Autodesk Inventor part; units mm, degrees
ref_plane "Work Plane1" through (-20.8033, -6.3, -5.9) normal (0, 0, 1) x (1, 0, 0)
ref_plane "YZ Plane" through (0, 0, 0) normal (1, 0, 0) x (0, 1, 0)
ref_plane "XZ Plane" through (0, 0, 0) normal (0, 1, 0) x (-1, 0, 0)
sketch "Sketch1" plane through (0, 0, 0) normal (0, 0, 1) x (1, 0, 0)
  line L0 (0.8467, -0.7217) -> (0.8467, 0.7217) construction
  line L1 (0.8467, 0.7217) -> (2.0967, 1.4434) construction
  line L2 (2.0967, 1.4434) -> (3.3467, 0.7217) construction
  line L3 (3.3467, 0.7217) -> (3.3467, -0.7217) construction
  line L4 (3.3467, -0.7217) -> (2.0967, -1.4434) construction
  line L5 (2.0967, -1.4434) -> (0.8467, -0.7217) construction
  circle A0 centre (2.0967, 0) radius 2.45 construction
  line L6 (4.8467, -1.5877) -> (3.4717, -2.3816) construction
  line L7 (15.0967, 3) -> (15.0967, -3) construction
  line L8 (-10.9033, 3) -> (-10.9033, -3) construction
  line L9 (-0.6533, 0) -> (-0.6533, 1.5877) construction
  circle A1 centre (2.0967, 0) radius 5
  circle A2 centre (2.0967, 0) radius 1.7
  line L10 (-10.9033, -3) -> (15.0967, -3)
  line L11 (-10.9033, 3) -> (15.0967, 3)
  circle A3 centre (2.0967, 0) radius 2.75
  circle A4 centre (2.0967, 0) radius 6.5
  point P0 (0.4719, -0.5)
  point P1 (3.7215, -0.5)
  dimension "d10" = 5.5
  dimension "d13" = 13
ref_plane "Work Plane1" through (-20.8033, -6.3, -5.9) normal (0, 0, 1) x (1, 0, 0)
extrude "Extrusion1" add sketch "Sketch1" against normal blind 5 contours A1 L10 L11 | A1 L11 A4 L10 | L11 A1 | A1 L11 A4 | L10 A4 A1 | A1 L10 | A1 L10 A4 L11
sketch "Sketch2" plane through (2.0967, 0, 0) normal (0, 0, 1) x (1, 0, 0)
  line L0 (-2, 1.5) -> (2, 1.5) construction
  arc A0 (2.5, 0) -> (2, 1.5) centre (0, 0) ccw construction
  arc A1 (-2, 1.5) -> (-2.5, 0) centre (0, 0) ccw construction
  line L1 (2, -1.5) -> (-2, -1.5) construction
  arc A2 (-2.5, 0) -> (2.5, 0) centre (0, 0) ccw construction
  line L2 (2.0248, 1.55) -> (-2.0248, 1.55) construction
  arc A3 (-2.0248, 1.55) -> (-2.55, 0) centre (0, 0) ccw construction
  arc A4 (-2.55, 0) -> (2.55, 0) centre (0, 0) ccw construction
  arc A5 (2.55, 0) -> (2.0248, 1.55) centre (0, 0) ccw construction
  line L3 (-2.0248, 1.55) -> (2.0248, 1.55) construction
  line L4 (-2.0248, 1.55) -> (2.0248, 1.55)
  line L5 (-2.0248, -1.55) -> (2.0248, -1.55)
  arc A6 (-2.0248, 1.55) -> (-2.0248, -1.55) centre (0, 0) ccw
  arc A7 (2.0248, -1.55) -> (2.0248, 1.55) centre (0, 0) ccw
  circle A8 centre (0, 0) radius 6.5
  point P0 (-2.0967, 0)
  dimension "d11" = 3.1
  dimension "d12" = 2.55
extrude "Extrusion2" add sketch "Sketch2" along normal blind 7
chamfer "Chamfer1" distance 1.2 angle 45 4 edges at (2.0967, 1.55, 7) (-0.4533, 0, 7) (2.0967, -1.55, 7) (4.6467, 0, 7)
sketch "Sketch3" plane through (0, 0, 0) normal (0, 1, 0) x (-1, 0, 0)
  line L0 (-4.6467, 0) -> (-4.6467, 5.8)
  line L1 (0.4533, 0) -> (0.4533, 5.8)
  line L2 (-8.5967, -5) -> (4.4033, -5)
  circle A0 centre (-2.0967, -2.5) radius 1.25
  line L3 (-8.5967, -5) -> (4.4033, -5)
  point P0 (0, 0)
  point P1 (-8.5967, 0)
  point P2 (4.4033, 0)
  dimension "d14" = 2.5
  dimension "d15" = 2.5
extrude "Extrusion3" cut sketch "Sketch3" against normal blind 10
pattern_circular "Circular Pattern1" count 2 over 360 about axis through (2.0967, 0, 0) along (0, 0, -1) of "Extrusion3"
sketch "Sketch4" plane through (0.0718, -1.55, 0) normal (0, 1, 0) x (1, 0, 0)
  line L0 (0, -5.8) -> (4.0497, -5.8)
  line L1 (-4.4752, -7) -> (8.5248, -7)
  line L2 (8.5248, 5) -> (-4.4752, 5)
  line L3 (4.0497, -5.8) -> (0, -5.8)
  line L4 (4.0497, 0) -> (4.0497, -5.8)
  line L5 (0, 0) -> (0, -5.8)
  circle A0 centre (2.0248, -2.0248) radius 2.0248
  line L6 (0, 0) -> (4.0497, 0)
  point P0 (-0.0718, 0)
  point P1 (3.2748, 2.5)
  point P2 (0.7748, 2.5)
hole "Hole1" at (2.0967, -1.55, 2.0248) direction (0, -1, 0) diameter 2.5 end through all both
properties part number "30_Coupling_Screw_28BYJ_M3_v2"
Geometry check sheet. Reference: the model listing, model coordinates, mm. A direction names the side the tool comes from. Give positions to 0.01 mm unless a question says otherwise; leave off trailing zeros. Loops run counter-clockwise (first coordinate to the right, second up) from the corner with the lowest first, then second, coordinate; pieces in that order, holes last.
(1) Section check A-A on y = 0. Record the cut outline in (x, z), then the cut area to 3 significant figures.
From the geometry:
outline: (-4.4, -5) - (-0.65, -5) - (-0.65, 0) - (-0.45, 0) - (-0.45, 5.8) - (-1.65, 7) - (-4.4, 7) - close; (4.65, 0) - (4.85, 0) - (4.85, -5) - (8.6, -5) - (8.6, 7) - (5.85, 7) - (4.65, 5.8) - close
area: 91.4 mm2
(2) Depth check by flat-ended pin: pin 1 Ø4 at (y, z) = (-3, -1.5) entering from +X; pin 2 Ø3 at (y, z) = (-4.5, 1) entering from +X; pin 3 Ø2 at (x, z) = (2, 2) entering from +Y; pin 4 Ø3 at (x, z) = (4.5, -1) entering from +Y. Enter the tip coordinate at first touch or a pass-through.
From the geometry:
pin 1: stops at x = 8.52
pin 2: stops at x = 7.86
pin 3: passes through
pin 4: stops at y = 6.44
(3) Release check for a two-part mould opening along Y. For faces 1 (the cylindrical face through (0.688, 6.345, 0.916)), 2 (the cylindrical face through (0.848, 4.446, -2.445)), 3 (the flat face through (2, -1.55, 4)) record: released by +Y, released by -Y, zero draft, split by the parting line, or undercut.
From the geometry:
face 1: split by the parting line
face 2: zero draft
face 3: undercut
(4) Section check D-D on x = 2.75. Count the separate pieces of the cut face and the enclosed holes in it, then the cut area to 3 significant figures.
From the geometry:
separate pieces: 6
enclosed holes: 0
area: 68.2 mm2
(5) Thickness scan on L1, parallel to Z at x = 1.5, y = -3; L2, parallel to X at y = 0.5, z = 6; L3, parallel to Z at x = 4, y = 2.25. Record the ranges inside material, lowest first.
From the geometry:
L1: z = -5 to -3.6, -1.4 to 0.93, 3.12 to 7
L2: x = -4.38 to -0.61, 4.8 to 8.58
L3: z = -5 to 6.5
(6) Section check B-B on z = -2.75. Record the cut outline in (x, y), then the cut area to 3 significant figures.
From the geometry:
outline: (0.87, -6.38) - (0.87, -2.46) arc R2.75 cw to (0.87, 2.46) - (0.87, 6.38) arc R6.5 ccw to start; (3.32, -6.38) arc R6.5 ccw to (3.32, 6.38) - (3.32, 2.46) arc R2.75 cw to (3.32, -2.46) - close
area: 90.3 mm2
(7) Set-up check for faces 4 (the cylindrical face through (4.647, 0.023, 2.859)), 5 (the flat face through (2, -2, 0)), 6 (the conical face through (-0.928, 0.035, 6.275)): record each of +Z, -Z, +X, -X, +Y, -Y from which the full face is reachable in a straight line by a thin tool's end or side.
From the geometry:
face 4: +Z, -Z
face 5: -Z
face 6: +Z
(8) Section check C-C on z = 5.5. Record the cut outline in (x, y).
From the geometry:
outline: circle Ø13 at (2.1, 0); hole (0.07, -1.55) - (4.12, -1.55) arc R2.55 ccw to (4.12, 1.55) - (0.07, 1.55) arc R2.55 ccw to start
